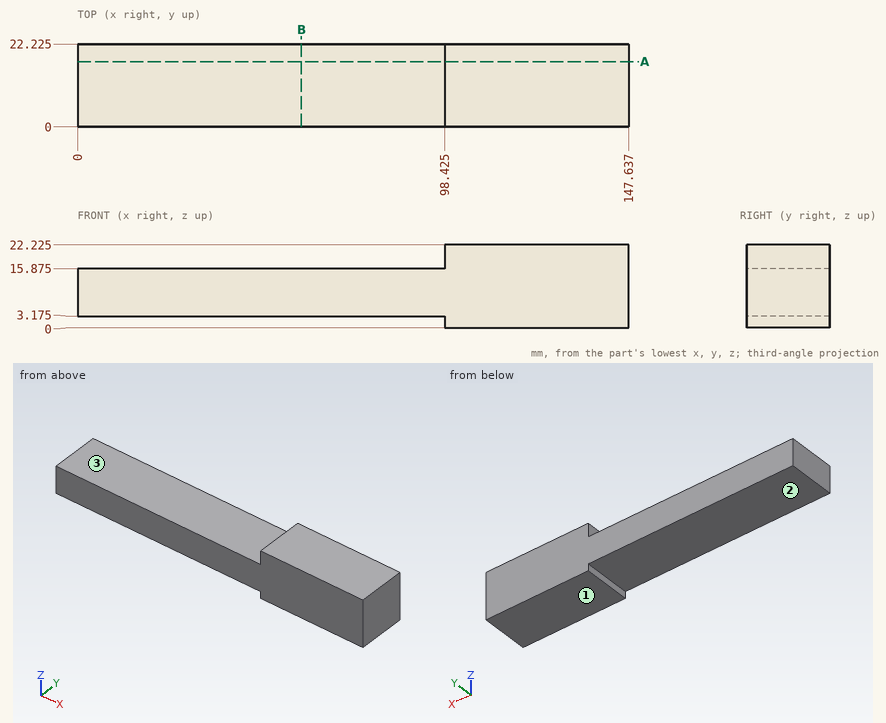
Here's the drawing with two shaded views (mm, measured from the low corner). I have some questions. A direction names the side the tool comes from. Round coordinates to 2 decimals unless told otherwise and drop trailing zeros. Write each loop counter-clockwise with the first axis right and the second up, starting at its lowest first coordinate (ties: lowest second). Pieces come first, ordered by that corner, then holes. Notation, with made-up numbers: M -16,88 L 10,88 A24 ccw 10,124 Z; hole C 19.5,-13 d8. An arc over 180 degrees is marked long. Answer in a Markdown table with one row per item. Add a question column.
Q1. Imagine slicing it at A-A (y = 17.5). Please give me the cut outline in (x, z) (1 decimal), then the cut area to 3 significant figures.
Q2. Imagine slicing it at B-B (x = 60). Please give me the cut outline in (y, z) (1 decimal), then the cut area to 3 significant figures.
Q3. On a 3-axis mill with a long thin cutter (end or side, diameter ignored), from which of +Z, -Z, +X, -X, +Y, -Y can I reach the whole of each face in a straight line? I mean the marked faces 1, 2 and 3. Say none if no direction works.
Q4. Will these pins go through, and if not, where does the flat tip stop? pin 1 Ø8 at (x, y) = (22, 19) entering from +Z (1 decimal); pin 2 Ø1 at (y, z) = (9, 18) entering from -X (1 decimal); pin 3 Ø1.5 at (x, y) = (66.5, 19.5) entering from -Z (1 decimal).
Q5. If I drill on line 1 (X direction, y = 18.75, z = 18) (1 decimal); line 2 (Z direction, x = 60.5, y = 5) (1 decimal), over which ranges is the centre line in solid material (lowest first)? Write a range as from..to.
Values:
| question | item | result |
|---|---|---|
| 1 | outline | M 0,3.2 L 98.4,3.2 L 98.4,0 L 147.6,0 L 147.6,22.2 L 98.4,22.2 L 98.4,15.9 L 0,15.9 Z |
| 1 | area | 2,340 mm^2 |
| 2 | outline | M 0,3.2 L 22.2,3.2 L 22.2,15.9 L 0,15.9 Z |
| 2 | area | 282 mm^2 |
| 3 | face 1 | -Z, +X, -X, +Y, -Y |
| 3 | face 2 | -Z, -X, +Y, -Y |
| 3 | face 3 | +Z, -X, +Y, -Y |
| 4 | pin 1 | z = 15.9 |
| 4 | pin 2 | x = 98.4 |
| 4 | pin 3 | z = 3.2 |
| 5 | line 1 | 98.4..147.6 |
| 5 | line 2 | 3.2..15.9 |
